Can you work these out from the drawing? Everything is in mm from the part's minimum corner. Coordinates: 2 decimals unless noted, no trailing zeros. Write each loop counter-clockwise with the first axis right and the second up, starting at its lowest first coordinate (ties: lowest second). Pieces come first, ordered by that corner, then holes. Notation, with made-up numbers: (28, 59) -> (58, 59) arc R13 ccw to (58, 73) -> close; hole circle Ø7 at (43, -24.5). An arc over 180 degrees is marked (long way). Answer as CSV lines item,"result". Start each with the question number.
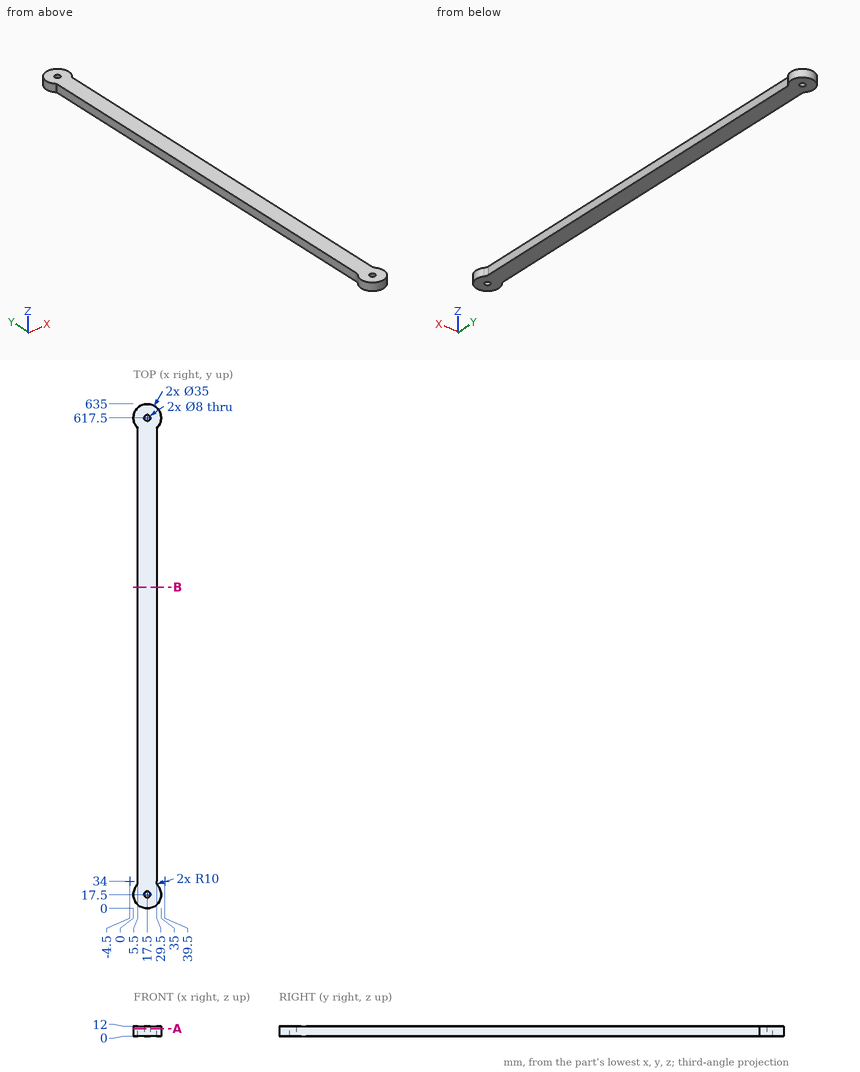
Q1. I need wall thicknesses on L1, parallel to Y at x = 17.5, z = 7.5; L2, parallel to Y at x = 16.5, z = 8.25; L3, parallel to X at y = 617.5, z = 3.25. Which ranges of each line are inside material? Lowest first, please.
Q2. Imagine slicing it at B-B (y = 404.5). Write out the boundary of the cut face in (x, z), then the cut area to 3 significant figures.
Q3. For pin 1 (4 mm diameter, centred on y = 419.5, z = 7.5, fed in from -X); pin 2 (2 mm diameter, centred on x = 27.5, z = 2, fed in from +Y); pin 3 (5 mm diameter, centred on y = 454, z = 7.5, fed in from +X), each with a flat end and sliding along its axis, tell me the tip position at first contact or that it passes through.
Q4. Imagine slicing it at A-A (z = 9.25). Write out the boundary of the cut face in (x, y).
Entries:
1,L1,"0 to 13.5, 21.5 to 613.5, 621.5 to 635"
1,L2,"0.03 to 13.63, 21.37 to 613.63, 621.37 to 634.97"
1,L3,"0 to 13.5, 21.5 to 35"
2,outline,"(5.5, 0) -> (29.5, 0) -> (29.5, 12) -> (5.5, 12) -> close"
2,area,"288 mm2"
3,pin 1,"x = 5.5"
3,pin 2,"y = 632.51"
3,pin 3,"x = 29.5"
4,outline,"(3.5, 28) arc R17.5 ccw (long way) to (31.5, 28) arc R10 cw to (29.5, 34) -> (29.5, 604.76) arc R17.5 ccw (long way) to (5.5, 604.76) -> (5.5, 34) arc R10 cw to start; hole circle Ø8 at (17.5, 17.5); hole circle Ø8 at (17.5, 617.5)"
